```python
from build123d import *

# Parameters (mm, degrees)
SKETCH1_W           = 110
SKETCH1_H           = 70
BOSS_EXTRUDE1_DEPTH = 6
SKETCH2_R           = 22.5
CUT_EXTRUDE1_DEPTH  = 3
SKETCH3_R           = 6.6
CUT_EXTRUDE2_DEPTH  = 3.2
SKETCH4_W           = 110
SKETCH4_H           = 70
SKETCH4_R           = 25
CUT_EXTRUDE3_DEPTH  = 3
SKETCH5_R           = 1.5
CUT_EXTRUDE4_DEPTH  = 77.389408912
CUT_EXTRUDE5_DEPTH  = 5
CUT_EXTRUDE6_DEPTH  = 11.5


with BuildPart() as part:
    # Sketch1 → Boss-Extrude1 (new body)
    with BuildSketch(Plane(origin=(0, 0, 0), x_dir=(1, 0, 0), z_dir=(0, 1, 0))):
        with Locations((-4.959349593, 12.235772358)):
            Rectangle(SKETCH1_W, SKETCH1_H)
    extrude(amount=BOSS_EXTRUDE1_DEPTH)

    # Sketch2 → Cut-Extrude1 (cut)
    with BuildSketch(Plane(origin=(0, 6, 0), x_dir=(1, 0, 0), z_dir=(0, 1, 0))):
        with Locations(Location((-4.959349593, 12.235772358, 0), (0, 0, 270))):
            Circle(SKETCH2_R)
    extrude(amount=-CUT_EXTRUDE1_DEPTH, mode=Mode.SUBTRACT)

    # Sketch3 → Cut-Extrude2 (cut)
    with BuildSketch(Plane(origin=(0, 3, 0), x_dir=(1, 0, 0), z_dir=(0, 1, 0))):
        with Locations(Location((-4.959349593, 12.235772358, 0), (0, 0, 270))):
            Circle(SKETCH3_R)
    extrude(amount=-CUT_EXTRUDE2_DEPTH, mode=Mode.SUBTRACT)

    # Sketch4 → Cut-Extrude3 (cut)
    with BuildSketch(Plane(origin=(0, 6, 0), x_dir=(1, 0, 0), z_dir=(0, 1, 0))):
        with Locations((-4.959349593, 12.235772358)):
            Rectangle(SKETCH4_W, SKETCH4_H)
        with Locations(Location((-4.959349593, 12.235772358, 0), (0, 0, 270))):
            Circle(SKETCH4_R, mode=Mode.SUBTRACT)
    extrude(amount=-CUT_EXTRUDE3_DEPTH, mode=Mode.SUBTRACT)

    # Sketch5 → Cut-Extrude4 (cut, through all)
    with BuildSketch(Plane(origin=(0, 3, 0), x_dir=(1, 0, 0), z_dir=(0, 1, 0))):
        with Locations(Location((-56.459349593, 43.735772358, 0), (0, 0, 270))):
            Circle(SKETCH5_R)
        with Locations(Location((-56.459349593, -19.264227642, 0), (0, 0, 270))):
            Circle(SKETCH5_R)
        with Locations(Location((46.540650407, -19.264227642, 0), (0, 0, 270))):
            Circle(SKETCH5_R)
        with Locations(Location((46.540650407, 43.735772358, 0), (0, 0, 270))):
            Circle(SKETCH5_R)
    extrude(amount=-CUT_EXTRUDE4_DEPTH, mode=Mode.SUBTRACT)

    # Sketch6 → Cut-Extrude5 (cut)
    with BuildSketch(Plane(origin=(0, 3, 0), x_dir=(1, 0, 0), z_dir=(0, 1, 0))):
        with BuildLine():
            Line((-16.640340857, 20.239524173), (-13.34062581, 17.978577332))
            ThreePointArc((-13.34062581, 17.978577332), (1.290813758, 20.245832163), (2.648826126, 5.502180284))
            Line((2.648826126, 5.502180284), (5.644170898, 2.851159782))
            ThreePointArc((5.644170898, 2.851159782), (3.751507991, 23.399399015), (-16.640340857, 20.239524173))
        make_face()
        with BuildLine():
            Line((-23.2771021, 20.239524173), (-19.611718907, 18.637973034))
            ThreePointArc((-19.611718907, 18.637973034), (-14.365152691, -0.69523565), (5.644170898, 0.267253101))
            Line((5.644170898, 0.267253101), (8.296708857, -2.726747963))
            ThreePointArc((8.296708857, -2.726747963), (-16.718074041, -3.930009385), (-23.2771021, 20.239524173))
        make_face()
    extrude(amount=-CUT_EXTRUDE5_DEPTH, mode=Mode.SUBTRACT)

    # Sketch7 → Cut-Extrude6 (cut)
    # profile 1 of 2: a face of its own
    with BuildSketch(Plane(origin=(0, 3, 0), x_dir=(1, 0, 0), z_dir=(0, 1, 0))):
        with BuildLine():
            Line((-54.989769689, 0.681181381), (-54.989769689, 24.493681381))
            Line((-54.989769689, 24.493681381), (-50.18147642, 24.493681381))
            add(Edge.make_bspline(
                [(-50.18147642, 24.493681381), (-49.763267768, 24.490670325), (-48.955290829, 24.484852979), (-47.787713285, 24.447968157), (-46.707416615, 24.382718738), (-45.71795377, 24.287676069), (-44.816608381, 24.170974179), (-44.00590428, 24.024694643), (-43.281649522, 23.851964412), (-42.836223506, 23.704698045), (-42.625586997, 23.635057583)],
                knots=[0, 0, 0, 0, 1.314313732, 2.53924729, 3.670748893, 4.714932338, 5.66265055, 6.526160246, 7.303039223, 8, 8, 8, 8], degree=3))
            add(Edge.make_bspline(
                [(-42.625586997, 23.635057583), (-42.350078145, 23.530073675), (-41.805308069, 23.322486546), (-41.029652467, 22.930898138), (-40.299456694, 22.487216143), (-39.610805012, 21.99085572), (-38.979427961, 21.427762563), (-38.38065995, 20.82185632), (-37.838995489, 20.151103505), (-37.34295869, 19.429414748), (-36.895721435, 18.665291678), (-36.506971093, 17.860190313), (-36.18411446, 17.018199309), (-35.916099829, 16.141660177), (-35.704873038, 15.228645535), (-35.560760252, 14.278092268), (-35.465707625, 13.293757068), (-35.456155061, 12.625820092), (-35.451308151, 12.286913052)],
                knots=[0, 0, 0, 0, 0.984719456, 1.947108742, 2.898477687, 3.838006223, 4.779231079, 5.722358779, 6.681677486, 7.655904652, 8.64651281, 9.637519902, 10.640069247, 11.656948941, 12.698408672, 13.768548281, 14.867775369, 16, 16, 16, 16], degree=3))
            add(Edge.make_bspline(
                [(-35.451308151, 12.286913052), (-35.455587376, 11.992582126), (-35.464020036, 11.412572294), (-35.539739131, 10.557765486), (-35.64979588, 9.728317795), (-35.820185869, 8.928179015), (-36.027031541, 8.150338818), (-36.292126927, 7.403087299), (-36.595807714, 6.679569596), (-36.94993278, 5.989568554), (-37.338698275, 5.335858468), (-37.755905135, 4.719621392), (-38.201108366, 4.149650687), (-38.678553297, 3.624220308), (-39.182070082, 3.144122355), (-39.71495526, 2.705346322), (-40.278583873, 2.316477619), (-40.870431469, 1.962235329), (-41.507763705, 1.653214696), (-42.202652366, 1.391753379), (-42.958060916, 1.175082657), (-43.772135159, 0.994305669), (-44.646281677, 0.850904735), (-45.581357498, 0.754794815), (-46.575925951, 0.689800755), (-47.258863452, 0.684110293), (-47.610375158, 0.681181381)],
                knots=[0, 0, 0, 0, 1.105936401, 2.179363191, 3.223086493, 4.248585256, 5.251745608, 6.245858792, 7.225916811, 8.198733463, 9.158002045, 10.082870192, 10.993790845, 11.873723703, 12.748670949, 13.606408763, 14.465103618, 15.319838547, 16.196477973, 17.123216899, 18.106603292, 19.147568657, 20.255746949, 21.433717677, 22.679120308, 24, 24, 24, 24], degree=3))
            Line((-47.610375158, 0.681181381), (-54.989769689, 0.681181381))
        make_face()
        with BuildLine():
            Line((-52.852750458, 3.123489074), (-50.119464701, 3.123489074))
            add(Edge.make_bspline(
                [(-50.119464701, 3.123489074), (-49.726705607, 3.125177015), (-48.971286032, 3.128423544), (-47.885041444, 3.15691148), (-46.89254055, 3.203461091), (-45.993642423, 3.268605816), (-45.188854597, 3.354797645), (-44.476495156, 3.450897429), (-43.858899202, 3.570622943), (-43.485182854, 3.679146434), (-43.312486035, 3.729295864)],
                knots=[0, 0, 0, 0, 1.375205317, 2.645023457, 3.804390687, 4.853969522, 5.800190428, 6.637939096, 7.370582563, 8, 8, 8, 8], degree=3))
            add(Edge.make_bspline(
                [(-43.312486035, 3.729295864), (-43.095123072, 3.805846645), (-42.665588855, 3.957119791), (-42.0472729, 4.233056736), (-41.470622565, 4.559914389), (-40.925588286, 4.923240575), (-40.419901576, 5.335849981), (-39.947569642, 5.788770459), (-39.509543458, 6.284307053), (-39.110348613, 6.821844724), (-38.753104615, 7.398037798), (-38.443737858, 8.007221648), (-38.172605116, 8.642721554), (-37.959798977, 9.314296365), (-37.793005449, 10.01594228), (-37.674863555, 10.74770866), (-37.601284804, 11.509458845), (-37.592702453, 12.027565262), (-37.588327381, 12.291683184)],
                knots=[0, 0, 0, 0, 0.998632004, 1.973411704, 2.929992603, 3.868527914, 4.809262121, 5.754881198, 6.702106254, 7.672490631, 8.653608572, 9.636854334, 10.631411391, 11.644891563, 12.686317036, 13.754757253, 14.855430412, 16, 16, 16, 16], degree=3))
            add(Edge.make_bspline(
                [(-37.588327381, 12.291683184), (-37.591819569, 12.570177041), (-37.598680001, 13.117280688), (-37.684910578, 13.920038812), (-37.810923303, 14.692112523), (-37.993148024, 15.43355346), (-38.225359897, 16.145808141), (-38.515155584, 16.824937309), (-38.846262405, 17.478113292), (-39.240211893, 18.090260316), (-39.671664412, 18.669197362), (-40.150485341, 19.199569198), (-40.669067425, 19.682583991), (-41.221754525, 20.125763958), (-41.824123004, 20.511279324), (-42.461982936, 20.856129779), (-43.144691878, 21.148791469), (-43.61966754, 21.304449446), (-43.861051239, 21.383555179)],
                knots=[0, 0, 0, 0, 1.122418816, 2.205001699, 3.251619955, 4.274784885, 5.280384055, 6.268708349, 7.249350384, 8.229342522, 9.199999885, 10.157847722, 11.105861043, 12.055065948, 13.010012805, 13.98527497, 14.976112212, 16, 16, 16, 16], degree=3))
            add(Edge.make_bspline(
                [(-43.861051239, 21.383555179), (-44.06074386, 21.438775876), (-44.485345162, 21.556190228), (-45.17821723, 21.684269995), (-45.958009586, 21.79723989), (-46.828184338, 21.892884765), (-47.787749569, 21.961514576), (-48.837443267, 22.013026556), (-49.977719148, 22.047769895), (-50.768175316, 22.050142349), (-51.178434052, 22.051373689)],
                knots=[0, 0, 0, 0, 0.674548936, 1.434276114, 2.292660221, 3.240891867, 4.284742987, 5.42552168, 6.663806718, 8, 8, 8, 8], degree=3))
            Line((-51.178434052, 22.051373689), (-52.852750458, 22.051373689))
            Line((-52.852750458, 22.051373689), (-52.852750458, 3.123489074))
        make_face(mode=Mode.SUBTRACT)
    # profile 2 of 2: a face of its own
    with BuildSketch(Plane(origin=(0, 3, 0), x_dir=(1, 0, 0), z_dir=(0, 1, 0))):
        Polygon((19.872381176, 0.938358716), (23.015898303, 24.750858716), (23.321186765, 24.750858716), (33.152429253, 5.212397178), (42.95982108, 24.750858716), (43.269879673, 24.750858716), (46.43247733, 0.938358716), (44.285917834, 0.938358716), (42.005794637, 18.07267362), (33.410016392, 0.938358716), (32.928233039, 0.938358716), (24.299063868, 18.110834678), (22.023710803, 0.938358716), align=None)
    extrude(amount=-CUT_EXTRUDE6_DEPTH, mode=Mode.SUBTRACT)


with BuildPart() as cut_extrude6_kept_piece:
    # of the separate pieces the step leaves, the one the design keeps (cut_extrude6_pieces_kept)
    add(part.part.solids().sort_by_distance((-59.959349593, 0, -47.235772358))[0])


solid = cut_extrude6_kept_piece.part
```
The model under review builds one solid part; all positions refer to its coordinate system, in mm. A direction names the side the tool comes from. Round coordinates to 2 decimals unless told otherwise and drop trailing zeros. Loops run counter-clockwise (first coordinate to the right, second up) from the corner with the lowest first, then second, coordinate; pieces in that order, holes last. Notation, with made-up numbers: (-16, 67.25) - (32, 67.25) arc R24 ccw to (32, 80.25) - close; hole circle Ø5 at (7, 34.25). An arc over 180 degrees is marked (long way). Use a Markdown table: item, result. Add a question column.
Q1. For probe 1 along X at (y, z) = (1, -22.5); probe 2 along Z at (x, y) = (-1, 1); probe 3 along Y at (x, z) = (-33.5, 1), list the stretches that pass through material, from the lowest coordinate up.
Q2. Machinability: for faces 5 (the face through (-15.01, 1.52, -19.12)), 6 (the face through (-27.3, 6, -16.1)), 7 (the face through (-10, 3, -18)), which of the approach directions +Z, -Z, +X, -X, +Y, -Y give a long, thin tool a straight path to every point of the face, cutting with its end or side? Answer none if there is none.
Q3. Add section B-B (z = -31.5). State the section outline as (x, y) points, plus the area to 3 significant figures.
Q4. Add section A-A (x = 38). State the section outline as (y, z) points, plus the area to 3 significant figures.
Q5. Insertion check: pin 1 Ø1.8 at (x, z) = (-56.46, 19.26) entering from -Y; pin 2 Ø4 at (x, z) = (46.54, -43.74) entering from -Y; pin 3 Ø5 at (x, z) = (46.54, 19.26) entering from +Y; pin 4 Ø1.5 at (x, y) = (9.5, 5) entering from +Z. Each pin has a flat end and moves straight along its axis. Give the tip position at first contact, or say it passes through.
Q6. Add section C-C (y = 4.75). State the section outline as (x, z) points.
Q7. The part is to be moulded in two halves that separate along X. For faces 1 (the face through (45.97, 1.52, -42.35)), 2 (the face through (-57.924, 1.521, 18.939)), 3 (the face through (-6, 1, 22.764)), 4 (the face through (2.55, 4.52, 11.61)), say which applies: pulls with the +X half, pulls with the -X half, needs draft (parallel to the pull), parting line crosses it, or undercut.
Q8. Add section D-D (z = 9). State the section outline as (x, y) points.
Worked answers:
| question | item | result |
|---|---|---|
| 1 | probe 1 | -59.96 to -54.99, -40.34 to -14.71, 4.8 to 22.72, 24.45 to 41.83, 43.57 to 50.04 |
| 1 | probe 2 | -47.24 to -25.83, -21.59 to -17.52, -6.96 to 3.26, 7.36 to 22.76 |
| 1 | probe 3 | 0 to 3 |
| 2 | face 5 | +Y, -Y |
| 2 | face 6 | +Z, -Z, +X, -X, +Y |
| 2 | face 7 | +Y |
| 3 | outline | (-59.96, 0) - (50.04, 0) - (50.04, 3) - (10.97, 3) - (10.97, 6) - (6.67, 6) - (6.67, 3) - (-16.58, 3) - (-16.58, 6) - (-20.89, 6) - (-20.89, 3) - (-59.96, 3) - close |
| 3 | area | 356 mm² |
| 4 | outline | (0, -47.24) - (3, -47.24) - (3, -14.87) - (0, -14.87) - close; (0, -10.09) - (3, -10.09) - (3, 22.76) - (0, 22.76) - close |
| 4 | area | 196 mm² |
| 5 | pin 1 | through |
| 5 | pin 2 | y = 0 |
| 5 | pin 3 | y = 3 |
| 5 | pin 4 | z = 8.67 |
| 6 | outline | circle Ø50 at (-4.96, -12.24); hole circle Ø45 at (-4.96, -12.24) |
| 7 | face 1 | undercut |
| 7 | face 2 | undercut |
| 7 | face 3 | needs draft |
| 7 | face 4 | parting line crosses it |
| 8 | outline | (-59.96, 0) - (50.04, 0) - (50.04, 3) - (8.23, 3) - (8.23, 6) - (2.48, 6) - (2.48, 3) - (-12.4, 3) - (-12.4, 6) - (-18.15, 6) - (-18.15, 3) - (-59.96, 3) - close |
